```python
from build123d import *

# Parameters (mm, degrees)
SKETCH1_R           = 8.3
BOSS_EXTRUDE1_DEPTH = 16.125
SKETCH2_R           = 5.1
BOSS_EXTRUDE2_DEPTH = 8
BOSS_EXTRUDE3_DEPTH = 18.6


with BuildPart() as part:
    # Sketch1 → Boss-Extrude1 (new body)
    with BuildSketch(Plane(origin=(0, 0, 0), x_dir=(1, 0, 0), z_dir=(0, 1, 0))):
        with Locations(Location((0, 0, 0), (0, 0, 270))):
            Circle(SKETCH1_R)
    extrude(amount=-BOSS_EXTRUDE1_DEPTH)

    # Sketch2 → Boss-Extrude2 (add)
    with BuildSketch(Plane(origin=(0, 0, 0), x_dir=(1, 0, 0), z_dir=(0, 1, 0))):
        with Locations(Location((0, 0, 0), (0, 0, 270))):
            Circle(SKETCH2_R)
    extrude(amount=BOSS_EXTRUDE2_DEPTH)

    # Sketch3 → Boss-Extrude3 (add)
    with BuildSketch(Plane.XZ.offset(16.125)):
        with BuildLine():
            Line((-6.05, -4.962673171), (-6.05, 4.962673171))
            ThreePointArc((-6.05, 4.962673171), (0, 7.825), (6.05, 4.962673171))
            Line((6.05, 4.962673171), (6.05, -4.962673171))
            ThreePointArc((6.05, -4.962673171), (0, -7.825), (-6.05, -4.962673171))
        make_face()
    extrude(amount=BOSS_EXTRUDE3_DEPTH)


solid = part.part
```
Geometry check sheet. Reference: the model listing, model coordinates, mm. A direction names the side the tool comes from. Give positions to 0.01 mm unless a question says otherwise; leave off trailing zeros. Order: outer loops, then holes, each group sorted by start corner. A loop starts at its lowest first (then second) coordinate and runs counter-clockwise, first axis right, second up.
1. Thickness scan on L1, parallel to Y at x = 4.5, z = 3.25 (3 decimals); L2, parallel to Y at x = -6.75, z = 1.25 (3 decimals); L3, parallel to X at y = 6, z = -0.25. Record the ranges inside material, lowest first.
2. Section check B-B, the plane x = 0. Enter the section's corners in (y, z) (3 decimals).
3. Access from +Z, -Z, +X, -X, +Y, -Y to the whole of each face (thin tool, end or side, straight path). Record for faces 1 (the face through (6.05, -25, 0)), 2 (the face through (0.097, -25.295, -7.824)), 3 (the face through (-6.05, -25, 0)), 4 (the face through (-4, 0, -4)).
4. Section check A-A, the plane z = 0. Enter the section's corners in (x, y) (3 decimals).
5. Section check C-C, the plane y = -17.5. Enter the section's corners in (x, z) (3 decimals), and give its area (3 significant figures).
6. Gauge pin test, flat ends, axial feed: pin 1 Ø5 at (y, z) = (-23, 1) entering from -X; pin 2 Ø1.5 at (y, z) = (-8, -2) entering from +X; pin 3 Ø2 at (x, y) = (3, -27.5) entering from +Z. Record the tip position at first contact, or that the pin passes through.
7. Section check D-D, the plane z = 6.5. Enter the section's corners in (x, y) (3 decimals), and give its area (3 significant figures).
Values follow:
1. L1: y = -34.725 to 0
1. L2: y = -16.125 to 0
1. L3: x = -5.09 to 5.09
2. outline: (-34.725, -7.825) - (-16.125, -7.825) - (-16.125, -8.3) - (0, -8.3) - (0, -5.1) - (8, -5.1) - (8, 5.1) - (0, 5.1) - (0, 8.3) - (-16.125, 8.3) - (-16.125, 7.825) - (-34.725, 7.825) - close
3. face 1: +Z, -Z, +X, -Y
3. face 2: -Z, -Y
3. face 3: +Z, -Z, -X, -Y
3. face 4: +Y
4. outline: (-8.3, -16.125) - (-6.05, -16.125) - (-6.05, -34.725) - (6.05, -34.725) - (6.05, -16.125) - (8.3, -16.125) - (8.3, 0) - (5.1, 0) - (5.1, 8) - (-5.1, 8) - (-5.1, 0) - (-8.3, 0) - close
5. outline: (-6.05, -4.963) arc R7.825 ccw to (6.05, -4.963) - (6.05, 4.963) arc R7.825 ccw to (-6.05, 4.963) - close
5. area: 168 mm2
6. pin 1: stops at x = -6.05
6. pin 2: stops at x = 8.21
6. pin 3: stops at z = 7.57
7. outline: (-5.161, -16.125) - (-4.357, -16.125) - (-4.357, -34.725) - (4.357, -34.725) - (4.357, -16.125) - (5.161, -16.125) - (5.161, 0) - (-5.161, 0) - close
7. area: 329 mm2
